Geometry check sheet. Reference: the model listing, model coordinates, mm. Face numbers are marked on the shaded views. Round coordinates to 2 decimals unless told otherwise and drop trailing zeros. Order: outer loops, then holes, each group sorted by start corner. A loop starts at its lowest first (then second) coordinate and runs counter-clockwise, first axis right, second up.
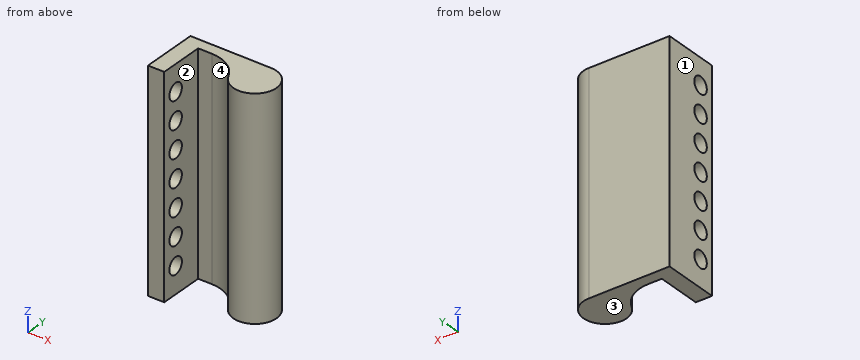
Autodesk Inventor part; units mm, degrees
ref_plane "YZ Plane" through (0, 0, 0) normal (1, 0, 0) x (0, 1, 0)
ref_plane "XZ Plane" through (0, 0, 0) normal (0, 1, 0) x (-1, 0, 0)
ref_plane "XY Plane" through (0, 0, 0) normal (0, 0, 1) x (1, 0, 0)
sketch "Sketch1" plane through (0, 0, 0) normal (1, 0, 0) x (0, 1, 0)
  line L0 (0, 0) -> (16.51, 0)
  line L1 (16.51, 0) -> (16.51, -63.5)
  line L2 (16.51, -63.5) -> (0, -63.5)
  line L3 (0, -63.5) -> (0, 0)
  circle A0 centre (4.445, -7.62) radius 2.4329
  circle A1 centre (4.445, -15.6185) radius 2.4329
  circle A2 centre (4.445, -23.6169) radius 2.4329
  circle A3 centre (4.445, -31.6154) radius 2.4329
  circle A4 centre (4.445, -39.6138) radius 2.4329
  circle A5 centre (4.445, -47.6123) radius 2.4329
  circle A6 centre (4.445, -55.6108) radius 2.4329
  dimension "d0" = 63.5
  dimension "d1" = 16.51
  dimension "d6" = 7.9985
  dimension "d11" = 7.62
extrude "Extrusion1" add sketch "Sketch1" along normal blind 4.7625
sketch "Sketch2" plane through (4.7625, 0, 0) normal (1, 0, 0) x (0, 0, -1)
  line L0 (63.5, 16.51) -> (0, 16.51)
  line L1 (63.5, 0) -> (63.5, 16.51)
  line L2 (0, 16.51) -> (63.5, 16.51)
  line L3 (63.5, 16.51) -> (63.5, 13.208)
  line L4 (63.5, 13.208) -> (0, 13.208)
  line L5 (0, 13.208) -> (0, 16.51)
  point P0 (0, 0)
  dimension "d14" = 3.302
extrude "Extrusion2" add sketch "Sketch2" along normal blind 1.016
sketch "Sketch3" plane through (0, 0, 0) normal (0, 0, 1) x (1, 0, 0)
  line L0 (5.7785, 16.51) -> (5.7785, 13.208)
  arc A0 (18.0184, 7.4246) -> (23.749, 16.51) centre (23.749, 10.16) ccw
  line L1 (0, 16.51) -> (0, 0)
  line L2 (5.7785, 16.51) -> (23.749, 16.51)
  line L3 (4.7625, 13.208) -> (5.7785, 13.208)
  line L4 (5.7785, 13.208) -> (8.8494, 13.208)
  arc A1 (18.0184, 7.4246) -> (8.8494, 13.208) centre (8.8494, 3.048) ccw
  point P0 (18.1783, 13.208)
  point P1 (9.5258, 13.208)
  dimension "d17" = 23.749
  dimension "d18" = 12.7
extrude "Extrusion3" add sketch "Sketch3" against normal blind 63.5
properties part number "knuckle plate original"
(1) Sectioned sample at D-D, the plane x = 3.5. Record the cut outline in (y, z) (1 decimal), and give its area (3 significant figures).
Returned:
outline: (0, -63.5) - (16.5, -63.5) - (16.5, 0) - (0, 0) - close; hole circle Ø4.9 at (4.4, -55.6); hole circle Ø4.9 at (4.4, -47.6); hole circle Ø4.9 at (4.4, -39.6); hole circle Ø4.9 at (4.4, -31.6); hole circle Ø4.9 at (4.4, -23.6); hole circle Ø4.9 at (4.4, -15.6); hole circle Ø4.9 at (4.4, -7.6)
area: 918 mm2
(2) Draft check along X on the marked faces 1, 2, 3 and 4. Enter one of: released by +X, released by -X, zero draft, split by the parting line, or undercut.
Returned:
face 1: released by -X
face 2: undercut
face 3: zero draft
face 4: undercut
(3) Sectioned sample at C-C, the plane z = -20. Record the cut outline in (x, y), and give its area (3 significant figures).
Returned:
outline: (0, 0) - (4.76, 0) - (4.76, 13.21) - (8.85, 13.21) arc R10.16 cw to (18.02, 7.42) arc R6.35 ccw (long way) to (23.75, 16.51) - (0, 16.51) - close
area: 268 mm2
(4) Material ranges on line 1 (X direction, y = 7.5, z = -38); line 2 (Y direction, x = 8, z = -33); line 3 (Y direction, x = 3, z = -39.5), recorded low to high.
Returned:
line 1: x = 0 to 4.76, 17.98 to 29.51
line 2: y = 13.21 to 16.51
line 3: y = 0 to 2.01, 6.88 to 16.51
(5) Sectioned sample at A-A, the plane z = -7.62. Record the cut outline in (x, y), and give its area (3 significant figures).
Returned:
outline: (0, 0) - (4.76, 0) - (4.76, 2.01) - (0, 2.01) - close; (0, 6.88) - (4.76, 6.88) - (4.76, 13.21) - (8.85, 13.21) arc R10.16 cw to (18.02, 7.42) arc R6.35 ccw (long way) to (23.75, 16.51) - (0, 16.51) - close
area: 244 mm2
(6) Depth check by flat-ended pin: P1, Ø4.5, axis at y = 4.44, z = -47.61, coming from the -X side; P2, Ø4, axis at y = 4.445, z = -7.62, coming from the +X side; P3, Ø3, axis at y = 4.44, z = -15.62, coming from the +X side. Enter the tip coordinate at first touch or a pass-through.
Returned:
P1: stops at x = 18.43
P2: stops at x = 28.9
P3: stops at x = 28.49
(7) Sectioned sample at B-B, the plane y = 9. Record the cut outline in (x, z).
Returned:
outline: (0, -63.5) - (4.76, -63.5) - (4.76, 0) - (0, 0) - close; (17.08, -63.5) - (29.99, -63.5) - (29.99, 0) - (17.08, 0) - close
